from build123d import *

# Parameters (mm, degrees)
SKETCH1_W                = 40
SKETCH1_H                = 35
SKETCH1_R                = 2.25
BOSS_EXTRUDE1_DEPTH      = 27
BOSS_EXTRUDE2_DEPTH      = 14
BOSS_EXTRUDE2_DEPTH_BACK = 54
SKETCH2_R                = 6
SKETCH3_R                = 12
BOSS_EXTRUDE3_DEPTH      = 3
BOSS_EXTRUDE4_DEPTH      = 8


with BuildPart() as part:
    # Sketch1 → Boss-Extrude1 (new body)
    with BuildSketch(Plane.YZ):
        Rectangle(SKETCH1_W, SKETCH1_H)
        with Locations(Location((-14, 12.5, 0), (0, 0, 270))):
            Circle(SKETCH1_R, mode=Mode.SUBTRACT)
        with Locations(Location((14, 12.5, 0), (0, 0, 270))):
            Circle(SKETCH1_R, mode=Mode.SUBTRACT)
    extrude(amount=BOSS_EXTRUDE1_DEPTH)

    # Sketch2 → Boss-Extrude2 (add, two sides: drawn at the far end of the back side and taken through both)
    with BuildSketch(Plane(origin=(0, 20, 0), x_dir=(-1, 0, 0), z_dir=(0, 1, 0)).offset(-BOSS_EXTRUDE2_DEPTH_BACK)):
        Polygon((-0.798294078, -2.5), (-7.149147039, 8.5), (-19.850852961, 8.5), (-26.201705922, -2.5), (-19.850852961, -13.5), (-7.149147039, -13.5), align=None)
        with Locations(Location((-13.5, -2.5, 0), (0, 0, 90))):
            Circle(SKETCH2_R, mode=Mode.SUBTRACT)
    extrude(amount=BOSS_EXTRUDE2_DEPTH + BOSS_EXTRUDE2_DEPTH_BACK)

    # Sketch3 → Boss-Extrude3 (add)
    with BuildSketch(Plane.XY.offset(17.5)):
        with Locations((13.5, 0)):
            Circle(SKETCH3_R)
    extrude(amount=BOSS_EXTRUDE3_DEPTH)

    # Sketch4 → Boss-Extrude4 (add)
    with BuildSketch(Plane.XY.offset(20.5)):
        Polygon((13.5, 6.363961031), (7.136038969, 0), (13.5, -6.363961031), (19.863961031, 0), align=None)
    extrude(amount=BOSS_EXTRUDE4_DEPTH)


solid = part.part
Part model, mm, in its own coordinate system. A direction names the side the tool comes from. Coordinates: 2 decimals unless noted, no trailing zeros. Loops run counter-clockwise (first coordinate to the right, second up) from the corner with the lowest first, then second, coordinate; pieces in that order, holes last. Notation, with made-up numbers: (85, 1.25) -> (119, 1.25) arc R14 ccw to (119, 5.25) -> close; hole circle Ø2 at (-21, -6.75). An arc over 180 degrees is marked (long way). Use a Markdown table: item, result. Add a question column.
Item 1: Band-saw the part on C-C on y = -25. Write the cut outline in (x, z).
Item 2: Flat gauge pins, fed straight in: P1, Ø4, axis at x = 14.5, y = -27.5, coming from the -Z side; P2, Ø8, axis at x = 7, y = 27, coming from the +Z side; P3, Ø1.5, axis at y = -27, z = -10, coming from the -X side; P4, Ø13.5, axis at x = 18, z = -5, coming from the -Y side. Where does each tip first touch, or does it go through?
Item 3: Which spindle directions (+Z, -Z, +X, -X, +Y, -Y) get a long thin tool onto all of the face, cutting with end or side? Do faces 4 (the cylindrical face through (1.51, 0.53, 18.98)), 5 (the cylindrical face through (7.643, -27.098, -3.801)), 6 (the flat face through (23.071, -27.098, -7.923)), 7 (the flat face through (10.363, 3.227, 24.444)). Say none if no direction does.
Item 4: Band-saw the part on B-B on z = 12.5. Write the cut outline in (x, y), plus the area to 3 significant figures.
Item 5: Pull direction X, two halves, no side cores. Call faces 1 (the flat face through (8, -34, 3)), 2 (the cylindrical face through (7.643, 26.902, -3.801)), 3 (the flat face through (3.929, -27.098, 2.923)): +X half, -X half, draft (parallel to the pull), parting line (faces both ways), or undercut.
Item 6: Band-saw the part on A-A on y = 14. Write the cut outline in (x, z), plus the area to 4 significant figures.
Item 7: Probe probe 1 along Y at (x, z) = (13.5, 12.5); probe 2 along Z at (x, y) = (13.5, 25); probe 3 along X at (y, z) = (-29.5, -2.5). List the from-to ranges inside material, lowest first.
Item 8: Band-saw the part on D-D on x = 18.5. Give the number of separate pieces and of enclosed holes in the cut face, plus the area to 3 significant figures.
Geometry says:
| question | item | result |
|---|---|---|
| 1 | outline | (0.8, -2.5) -> (7.15, -13.5) -> (19.85, -13.5) -> (26.2, -2.5) -> (19.85, 8.5) -> (7.15, 8.5) -> close; hole circle Ø12 at (13.5, -2.5) |
| 2 | P1 | z = -13.5 |
| 2 | P2 | z = 8.5 |
| 2 | P3 | x = 4.7 |
| 2 | P4 | y = -34 |
| 3 | face 4 | +Z |
| 3 | face 5 | -Y |
| 3 | face 6 | -Z, +X, -Y |
| 3 | face 7 | +Z, -X, +Y |
| 4 | outline | (0, -20) -> (27, -20) -> (27, -16.25) -> (0, -16.25) -> close; (0, -11.75) -> (27, -11.75) -> (27, 11.75) -> (0, 11.75) -> close; (0, 16.25) -> (27, 16.25) -> (27, 20) -> (0, 20) -> close |
| 4 | area | 837 mm² |
| 5 | face 1 | draft |
| 5 | face 2 | undercut |
| 5 | face 3 | -X half |
| 6 | outline | (0, -17.5) -> (27, -17.5) -> (27, 10.25) -> (0, 10.25) -> close; (0, 14.75) -> (27, 14.75) -> (27, 17.5) -> (0, 17.5) -> close |
| 6 | area | 823.5 mm² |
| 7 | probe 1 | -20 to -16.25, -11.75 to 11.75, 16.25 to 20 |
| 7 | probe 2 | -13.5 to -8.5, 3.5 to 8.5 |
| 7 | probe 3 | 0.8 to 7.5, 19.5 to 26.2 |
| 8 | separate pieces | 1 |
| 8 | enclosed holes | 2 |
| 8 | area | 1,890 mm² |
